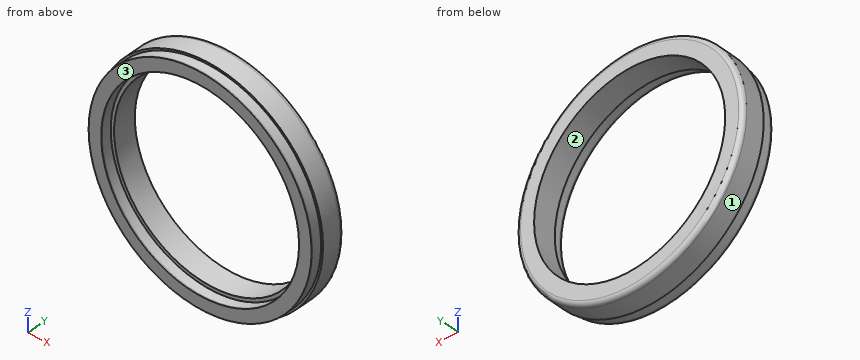
```python
from build123d import *

# Parameters (mm, degrees)
F0_R     = 33.909
F0_R_2   = 28.575
F1_DEPTH = 9.652
F2_R     = 33.3375
F2_R_2   = 29.591
F3_DEPTH = 4.699
F4_R     = 1.27
F5_DEPTH = 1.5367
F6_DEPTH = 2.7686
F7_DEPTH = 2.7813


with BuildPart() as f1:
    # F0 (on Front) → F1 (new body)
    with BuildSketch(Plane.XZ):
        Circle(F0_R)
        Circle(F0_R_2, mode=Mode.SUBTRACT)
    extrude(amount=F1_DEPTH)

    # F2 (on face) → F3 (join)
    with BuildSketch(Plane.XZ.offset(9.652)):
        Circle(F2_R)
        Circle(F2_R_2, mode=Mode.SUBTRACT)
    extrude(amount=F3_DEPTH)

    # F4
    f4_edges = [f1.edges().sort_by_distance(p)[0] for p in [
        (-33.909, 0, 0),
    ]]
    fillet(f4_edges, radius=F4_R)

    # F5 (cut): a face of the model
    f5_faces = [f1.faces().sort_by_distance(p)[0] for p in [
        (-32.3945731073, -14.351, 0),
    ]]
    extrude(f5_faces, amount=-F5_DEPTH, mode=Mode.SUBTRACT)

    # F6 (cut): a face of the model
    f6_faces = [f1.faces().sort_by_distance(p)[0] for p in [
        (-32.3945731073, -12.8143, 0),
    ]]
    extrude(f6_faces, amount=-F6_DEPTH, mode=Mode.SUBTRACT)

    # F7 (cut): faces of the model
    f7_faces = [f1.faces().sort_by_distance(p)[0] for p in [
        (-33.8130908646, -9.652, 0),
        (-28.7540401295, -9.652, 0),
    ]]
    extrude(f7_faces, amount=-F7_DEPTH, mode=Mode.SUBTRACT)


solid = f1.part
```
Source: CAD feature listing. Evaluate the final solid. Frame: model axes, mm. Face numbers are marked on the shaded views. Give positions to 0.01 mm unless a question says otherwise; leave off trailing zeros. Write each loop counter-clockwise with the first axis right and the second up, starting at its lowest first coordinate (ties: lowest second). Pieces come first, ordered by that corner, then holes.
1. Section query B-B (x = 0). Return the cut outline in (y, z) (1 decimal).
2. Material intervals for line 1 along X through (y, z) = (-4.75, 1); line 2 along Z through (x, y) = (0, -8.45); line 3 along X through (y, z) = (-4.25, -16.5), sorted ascending.
3. Section query A-A (z = 0). Return the cut outline in (x, y) (1 decimal).
4. Pull-direction query (Z, two-part tool) for the marked faces 1, 2 and 3; classes: +Z half, -Z half, draft (parallel to the pull), parting line (faces both ways), or undercut.
5. First-contact query: pin 1 (4 mm diameter, centred on x = 6.5, y = -7.5, fed in from +Z); pin 2 (1.5 mm diameter, centred on x = -8, y = -9, fed in from -Z); pin 3 (1 mm diameter, centred on y = -8, z = -19, fed in from -X). Flat tips, straight axial feed; report the tip coordinate or a pass-through.
Output values:
1. outline: (-10, -33.3) - (-6.9, -33.3) - (-6.9, -33.9) - (-1.3, -33.9) arc R1.3 ccw to (0, -32.6) - (0, -28.6) - (-6.9, -28.6) - (-6.9, -29.6) - (-10, -29.6) - close; (-10, 29.6) - (-6.9, 29.6) - (-6.9, 28.6) - (0, 28.6) - (0, 32.6) arc R1.3 ccw to (-1.3, 33.9) - (-6.9, 33.9) - (-6.9, 33.3) - (-10, 33.3) - close
2. line 1: x = -33.89 to -28.56, 28.56 to 33.89
2. line 2: z = -33.34 to -29.59, 29.59 to 33.34
2. line 3: x = -29.62 to -23.33, 23.33 to 29.62
3. outline: (-33.9, -6.9) - (-33.3, -6.9) - (-33.3, -10) - (-29.6, -10) - (-29.6, -6.9) - (-28.6, -6.9) - (-28.6, 0) - (-32.6, 0) arc R1.3 ccw to (-33.9, -1.3) - close; (28.6, -6.9) - (29.6, -6.9) - (29.6, -10) - (33.3, -10) - (33.3, -6.9) - (33.9, -6.9) - (33.9, -1.3) arc R1.3 ccw to (32.6, 0) - (28.6, 0) - close
4. face 1: parting line
4. face 2: undercut
4. face 3: draft
5. pin 1: stops at z = 33.6
5. pin 2: stops at z = -32.54
5. pin 3: stops at x = -27.73
